Geometry check sheet. Reference: drawing and pictorial views, mm from the part's lowest x, y, z. A direction names the side the tool comes from. Coordinates: 2 decimals unless noted, no trailing zeros. Loops run counter-clockwise (first coordinate to the right, second up) from the corner with the lowest first, then second, coordinate; pieces in that order, holes last. Notation, with made-up numbers: (78, 8.5) -> (88, 8.5) arc R17 ccw to (88, 23.5) -> close; hole circle Ø5 at (51, -29.5). An arc over 180 degrees is marked (long way). Answer as a JSON object with one key per item and string values. Group by question number.
Q1. Gauge pin test, flat ends, axial feed: pin 1 Ø5 at (x, z) = (3, 19.5) entering from +Y; pin 2 Ø3 at (x, z) = (4.5, 7.5) entering from -Y (1 decimal); pin 3 Ø12 at (y, z) = (2, 21) entering from -X. Record the tip position at first contact, or that the pin passes through.
Q2. Cross-section at C-C on z = 14.5. Record the boundary of the cut face in (x, y).
Q3. Scan lines: L1, parallel to X at y = 10, z = 3.5; L2, parallel to Z at x = 5, y = 5.75; L3, parallel to Z at x = 9.5, y = 2.5. Record each from-to range of solid material in increasing order.
Q4. Set-up check for the marked faces 1, 2 and 3: record each of +Z, -Z, +X, -X, +Y, -Y from which the full face is reachable in a straight line by a thin tool's end or side.
Q5. Cross-section at B-B on x = 8. Record the boundary of the cut face in (y, z).
Q6. Cross-section at A-A on y = 10. Record the boundary of the cut face in (x, z).
Q7. Cross-section at D-D on y = 13.5. Record the boundary of the cut face in (x, z), and give its area (3 significant figures).
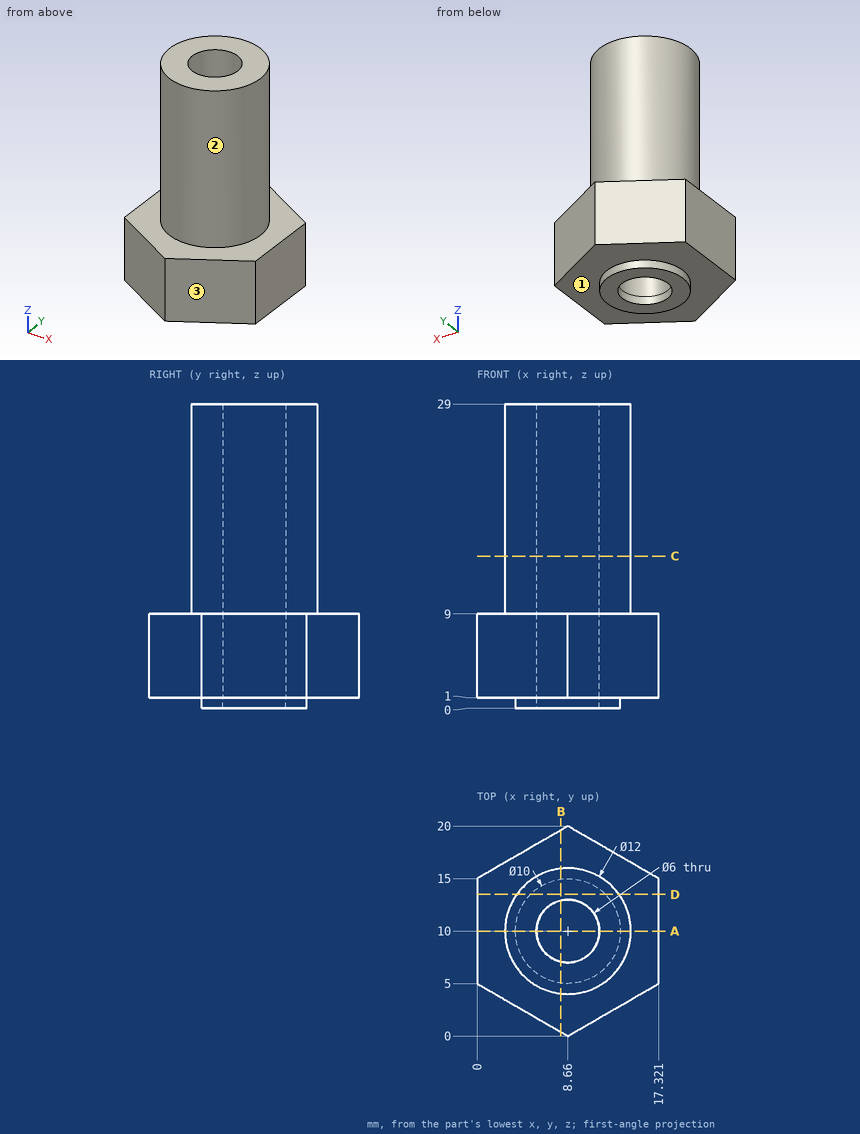
Computed values:
{
 "1": {"pin 1": "stops at y = 15.1", "pin 2": "stops at y = 1.5", "pin 3": "stops at x = 3"},
 "2": {"outline": "circle Ø12 at (8.66, 10); hole circle Ø6 at (8.66, 10)"},
 "3": {"L1": "x = 0 to 5.66, 11.66 to 17.32", "L2": "z = 1 to 29", "L3": "z = 1 to 9"},
 "4": {"face 1": "-Z", "face 2": "+Z", "face 3": "+Z, -Z, +X, -Y"},
 "5": {"outline": "(0.38, 1) -> (5.04, 1) -> (5.04, 0) -> (7.07, 0) -> (7.07, 29) -> (4.04, 29) -> (4.04, 9) -> (0.38, 9) -> close; (12.93, 0) -> (14.96, 0) -> (14.96, 1) -> (19.62, 1) -> (19.62, 9) -> (15.96, 9) -> (15.96, 29) -> (12.93, 29) -> close"},
 "6": {"outline": "(0, 1) -> (3.66, 1) -> (3.66, 0) -> (5.66, 0) -> (5.66, 29) -> (2.66, 29) -> (2.66, 9) -> (0, 9) -> close; (11.66, 0) -> (13.66, 0) -> (13.66, 1) -> (17.32, 1) -> (17.32, 9) -> (14.66, 9) -> (14.66, 29) -> (11.66, 29) -> close"},
 "7": {"outline": "(0, 1) -> (5.09, 1) -> (5.09, 0) -> (12.23, 0) -> (12.23, 1) -> (17.32, 1) -> (17.32, 9) -> (13.53, 9) -> (13.53, 29) -> (3.79, 29) -> (3.79, 9) -> (0, 9) -> close", "area": "341 mm²"}
}
